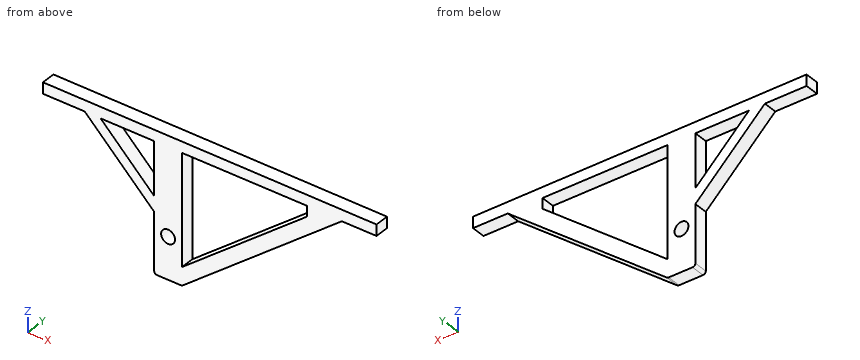
```python
from build123d import *

# Parameters (mm, degrees)
SKETCH1_R           = 6.35
BOSS_EXTRUDE1_DEPTH = 12.7


with BuildPart() as part:
    # Sketch1 → Boss-Extrude1 (new body)
    with BuildSketch(Plane(origin=(0, 0, 0), x_dir=(1, 0, 0), z_dir=(0, 1, 0))):
        with BuildLine():
            Line((171.45, 10.16), (26.09574153, 126.443406776))
            ThreePointArc((26.09574153, 126.443406776), (25.34977374, 126.856815931), (24.509016109, 127))
            Line((24.509016109, 127), (2.54, 127))
            ThreePointArc((2.54, 127), (0.743948776, 126.256051224), (0, 124.46))
            Line((0, 124.46), (0, 72.055027479))
            Line((0, 72.055027479), (-63.5, 9.332908944))
            Line((-63.5, 9.332908944), (-101.6, 9.332908944))
            Line((-101.6, 9.332908944), (-101.6, -0.827091056))
            Line((-101.6, -0.827091056), (203.2, 0))
            Line((203.2, 0), (203.2, 10.16))
            Line((203.2, 10.16), (171.45, 10.16))
        make_face()
        with Locations(Location((12.7, 88.9, 0), (0, 0, 90))):
            Circle(SKETCH1_R, mode=Mode.SUBTRACT)
        Polygon((0, 9.525), (0, 58.085027479), (-48.962001116, 9.525), align=None, mode=Mode.SUBTRACT)
        Polygon((25.4, 9.525), (25.4, 110.49), (139.7, 19.05), (139.7, 9.525), align=None, mode=Mode.SUBTRACT)
    extrude(amount=BOSS_EXTRUDE1_DEPTH)


solid = part.part
```
Could you check a few things on this model? Use its own coordinates, in mm. Round coordinates to 2 decimals unless told otherwise and drop trailing zeros. Loops run counter-clockwise (first coordinate to the right, second up) from the corner with the lowest first, then second, coordinate; pieces in that order, holes last.
Q1. I want a section at C-C (z = -88.9). Give the number of separate pieces and of enclosed holes in the cut face, and give its area (3 significant figures).
Q2. Please list where these lines run through material, in increasing order: L1, parallel to X at y = 4.25, z = -22.5 (1 decimal); L2, parallel to X at y = 4.75, z = -14.5 (3 decimals); L3, parallel to Z at x = 16, y = 7.75.
Q3. I want a section at A-A (x = 31). Write out the boundary of the cut face in (y, z) (3 decimals).
Q4. I want a section at D-D (z = -102.5). Write out the boundary of the cut face in (x, y) (1 decimal).
Q5. For P1, Ø3, axis at x = 81.5, y = 11, coming from the +Z side; P2, Ø1, axis at x = 27.5, y = 10.5, coming from the +Z side; P3, Ø4, axis at y = 8.5, z = -53.5, coming from the +X side (3 decimals); P4, Ø14.5, axis at x = 12.7, z = -88.9, coming from the +Y side, each with a flat end and sliding along its axis, tell me the tip position at first contact or that it passes through.
Q6. I want a section at B-B (y = 2). Write out the boundary of the cut face in (x, z) (3 decimals), and give its area (3 significant figures).
Answer below:
1. separate pieces: 3
1. enclosed holes: 0
1. area: 423 mm2
2. L1: x = -50.2 to -35.9, 0 to 25.4, 135.4 to 156
2. L2: x = -58.269 to -43.946, 0 to 25.4, 139.7 to 166.025
2. L3: z = -127 to -94.33, -83.47 to 0.51
3. outline: (0, -122.52) - (12.7, -122.52) - (12.7, -106.01) - (0, -106.01) - close; (0, -9.525) - (12.7, -9.525) - (12.7, 0.467) - (0, 0.467) - close
4. outline: (0, 0) - (25.4, 0) - (25.4, 12.7) - (0, 12.7) - close; (35.4, 0) - (56, 0) - (56, 12.7) - (35.4, 12.7) - close
5. P1: stops at z = 0.33
5. P2: stops at z = 0.48
5. P3: stops at x = 119.775
5. P4: stops at y = 12.7
6. outline: (-101.6, -9.333) - (-63.5, -9.333) - (0, -72.055) - (0, -124.46) arc R2.54 ccw to (2.54, -127) - (24.509, -127) arc R2.54 ccw to (26.096, -126.443) - (171.45, -10.16) - (203.2, -10.16) - (203.2, 0) - (-101.6, 0.827) - close; hole (-48.962, -9.525) - (0, -58.085) - (0, -9.525) - close; hole circle Ø12.7 at (12.7, -88.9); hole (25.4, -110.49) - (139.7, -19.05) - (139.7, -9.525) - (25.4, -9.525) - close
6. area: 9,000 mm2
